The model under review builds one solid part; all positions refer to its coordinate system, in mm. A direction names the side the tool comes from. Round coordinates to 2 decimals unless told otherwise and drop trailing zeros. Loops run counter-clockwise (first coordinate to the right, second up) from the corner with the lowest first, then second, coordinate; pieces in that order, holes last. Notation, with made-up numbers: M 63.25,74.25 L 88.25,74.25 A26 ccw 88.25,109.25 Z; hole C -3,67 d10. An arc over 180 degrees is marked long. Answer as a JSON object with one key per item and string values. Group by question number.
Item 1: To check wall thickness, follow line 1 (Z direction, x = 0, y = 17.5); line 2 (X direction, y = -32.5, z = 57) (3 decimals). State the ranges of each line that lie inside material, in increasing order.
Item 2: Consider section B-B (x = 0). Give the boundary of the cut face in (y, z).
Item 3: Consider section A-A (z = 71.5). Give the boundary of the cut face in (x, y) (3 decimals), and give its area (3 significant figures).
Item 4: Insertion check: P1, Ø5, axis at x = -24.5, y = -33.5, coming from the -Z side; P2, Ø7.5, axis at y = 0, z = 0, coming from the +X side; P3, Ø5, axis at x = 20, z = 38.5, coming from the -Y side; P4, Ø3, axis at x = -19.5, z = 12.5, coming from the -Y side. Each pin has a flat end and moves straight along its axis. Give the tip position at first contact, or say it passes through.
Item 5: The part is to be moulded in two halves that separate along Y. For faces 4 (the face through (-27.46, -90.15, 74.99)), 5 (the face through (27.46, -90.15, 74.99)), 6 (the face through (27.46, -78.11, 93.64)), 7 (the face through (32.544, -66, 72)), say which applies: +Y half, -Y half, draft (parallel to the pull), parting line (faces both ways), or undercut.
Item 6: Consider section C-C (y = 0). Give the boundary of the cut face in (x, z) (3 decimals), and give its area (3 significant figures).
Item 7: Tool access review of faces 1 (the face through (-0.46, -6.21, 1.38)), 2 (the face through (0.46, -11.97, -6.23)), 3 (the face through (10.265, 15.189, 4.256)): name each direction out of +Z, -Z, +X, -X, +Y, -Y from which nothing blocks a thin tool from reaching the whole face with its end or side.
```python
from build123d import *

# Parameters (mm, degrees)
SKETCH2_R           = 13.49375
SKETCH2_R_2         = 6.3627
BOSS_EXTRUDE1_DEPTH = 32.54375
BOSS_EXTRUDE2_REACH = 35.337
SKETCH3_R           = 11.1125
SKETCH3_R_2         = 3.571875
CUT_EXTRUDE1_REACH  = 35.338
SKETCH3_2_R         = 3.571875
SKETCH4_R           = 13.49375
SKETCH4_R_2         = 6.3627
SKETCH4_R_3         = 5.159375
BOSS_EXTRUDE3_DEPTH = 10.31875
BOSS_EXTRUDE4_REACH = 67.088
SKETCH4_3_R         = 5.159375


with BuildPart() as part:
    # Sketch2 → Boss-Extrude1 (new body, symmetric)
    with BuildSketch(Plane(origin=(0, 0, 0), x_dir=(0, 0, -1), z_dir=(1, 0, 0))):
        Circle(SKETCH2_R)
        Circle(SKETCH2_R_2, mode=Mode.SUBTRACT)
    extrude(amount=BOSS_EXTRUDE1_DEPTH, both=True)

    # Sketch3 → Boss-Extrude2 (add, up to next)
    with BuildSketch(Plane(origin=(0, 19.84375, 0), x_dir=(1, 0, 0), z_dir=(0, 1, 0)), mode=Mode.PRIVATE) as boss_extrude2_sk1:
        Circle(SKETCH3_R)
        Circle(SKETCH3_R_2, mode=Mode.SUBTRACT)
    boss_extrude2_tool1 = extrude(boss_extrude2_sk1.sketch, amount=-BOSS_EXTRUDE2_REACH, mode=Mode.PRIVATE) - part.part
    add(boss_extrude2_tool1.solids().sort_by_distance((-10.798191, 19.84375, 0))[0])

    # Sketch3<2> → Cut-Extrude1 (cut, up to next)
    with BuildSketch(Plane(origin=(0, 19.84375, 0), x_dir=(1, 0, 0), z_dir=(0, 1, 0)), mode=Mode.PRIVATE) as cut_extrude1_sk1:
        Circle(SKETCH3_2_R)
    cut_extrude1_tool1 = extrude(cut_extrude1_sk1.sketch, amount=-CUT_EXTRUDE1_REACH, mode=Mode.PRIVATE) & part.part
    add(cut_extrude1_tool1.solids().sort_by_distance((0, 19.84375, 0))[0], mode=Mode.SUBTRACT)

    # Sketch4 → Boss-Extrude3 (add)
    with BuildSketch(Plane(origin=(32.54375, 0, 0), x_dir=(0, 0, -1), z_dir=(1, 0, 0))):
        with BuildLine():
            ThreePointArc((0, -13.49375), (-13.49375, 0), (0, 13.49375))
            ThreePointArc((0, 13.49375), (-93.6625, -80.16875), (0, -173.83125))
            ThreePointArc((0, -173.83125), (-5.159375, -168.671875), (0, -163.5125))
            ThreePointArc((0, -163.5125), (-75.009375, -88.503125), (0, -13.49375))
        make_face()
        Circle(SKETCH4_R)
        Circle(SKETCH4_R_2, mode=Mode.SUBTRACT)
        with Locations((0, -168.671875)):
            Circle(SKETCH4_R_3)
    boss_extrude3 = extrude(amount=-BOSS_EXTRUDE3_DEPTH)

    # Mirror1: Boss-Extrude3 across plane
    add(boss_extrude3.mirror(Plane(origin=(0, 0, 0), x_dir=(0, 0, 1), z_dir=(1, 0, 0))))

    # Sketch4<3> → Boss-Extrude4 (add, up to next)
    with BuildSketch(Plane(origin=(32.54375, 0, 0), x_dir=(0, 0, -1), z_dir=(1, 0, 0)), mode=Mode.PRIVATE) as boss_extrude4_sk1:
        with Locations((0, -168.671875)):
            Circle(SKETCH4_3_R)
    boss_extrude4_tool1 = extrude(boss_extrude4_sk1.sketch, amount=-BOSS_EXTRUDE4_REACH, mode=Mode.PRIVATE) - part.part
    add(boss_extrude4_tool1.solids().sort_by_distance((32.54375, -168.671875, 0))[0])


solid = part.part
```
Geometry results:
{
 "1": {"line 1": "z = -11.11 to -3.57, 3.57 to 11.11", "line 2": "x = -32.544 to -22.225, 22.225 to 32.544"},
 "2": {"outline": "C -168.67,0 d10.32; M 5.27,-3.57 A6.36 cw long 5.27,3.57 L 19.84,3.57 L 19.84,11.11 L 7.65,11.11 A13.49 ccw long 7.65,-11.11 L 19.84,-11.11 L 19.84,-3.57 Z"},
 "3": {"outline": "M -32.544,-140.67 L -22.225,-140.67 L -22.225,-111.178 L -32.544,-111.178 Z; M -32.544,-65.828 L -22.225,-65.828 L -22.225,-19.667 L -32.544,-19.667 Z; M 22.225,-140.67 L 32.544,-140.67 L 32.544,-111.178 L 22.225,-111.178 Z; M 22.225,-65.828 L 32.544,-65.828 L 32.544,-19.667 L 22.225,-19.667 Z", "area": "1,560 mm^2"},
 "4": {"P1": "stops at z = 48.16", "P2": "passes through", "P3": "stops at y = -166.06", "P4": "stops at y = -7.82"},
 "5": {"face 4": "undercut", "face 5": "undercut", "face 6": "parting line", "face 7": "draft"},
 "6": {"outline": "M -32.544,-13.494 L 32.544,-13.494 L 32.544,-6.363 L -32.544,-6.363 Z; M -32.544,6.363 L 32.544,6.363 L 32.544,48.432 L 22.225,48.432 L 22.225,13.494 L -22.225,13.494 L -22.225,48.432 L -32.544,48.432 Z", "area": "1,650 mm^2"},
 "7": {"face 1": "+X, -X", "face 2": "none", "face 3": "+Y"}
}
